Here's the drawing with two shaded views (mm, measured from the low corner). I have some questions. Coordinates: 2 decimals unless noted, no trailing zeros. Write each loop counter-clockwise with the first axis right and the second up, starting at its lowest first coordinate (ties: lowest second). Pieces come first, ordered by that corner, then holes. Notation, with made-up numbers: M -37.75,79.25 L 15.25,79.25 A16 ccw 15.25,87.25 Z; hole C -17.75,51 d5. An arc over 180 degrees is marked long. Answer as CSV lines item,"result". Start each with the question number.
Item 1: Suppose I cut it at C-C, the plane z = 7.75. Write out the boundary of the cut face in (x, y).
Item 2: Suppose I cut it at A-A, the plane x = 27.35. Write out the boundary of the cut face in (y, z).
Item 3: If I drill on line 1 along X through (y, z) = (0.5, 2.5) (1 decimal); line 2 along X through (y, z) = (0.35, 2); line 3 along X through (y, z) = (0.1, 6.25) (1 decimal), over which ranges is the centre line in solid material (lowest first)? Write a range as [from, to].
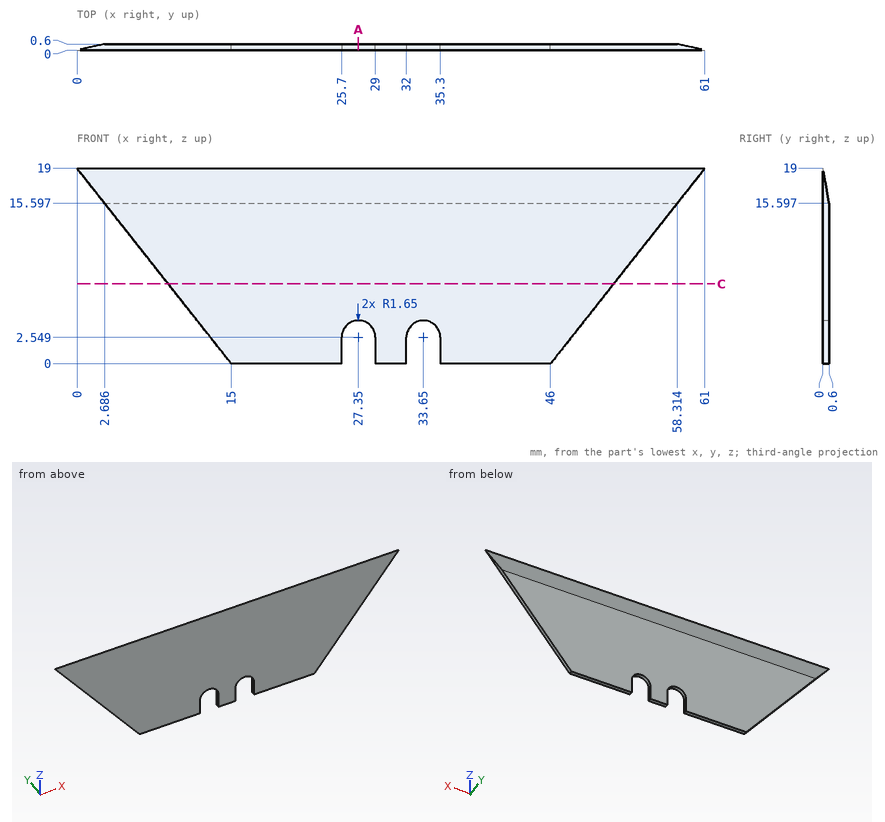
Ans:
1,outline,"M 8.88,0 L 52.12,0 L 52.12,0.6 L 8.88,0.6 Z"
2,outline,"M 0,4.2 L 0.6,4.2 L 0.6,15.6 L 0,19 Z"
3,line 1,"x = [13, 25.7], [29, 32], [35.3, 48]"
3,line 2,"x = [13.42, 25.7], [29, 32], [35.3, 47.58]"
3,line 3,"x = [10.1, 50.9]"
